Job drawing, mm, ordinate dimensions from the low corner. One solid piece. Round coordinates to 2 decimals unless told otherwise and drop trailing zeros. Write each loop counter-clockwise with the first axis right and the second up, starting at its lowest first coordinate (ties: lowest second). Pieces come first, ordered by that corner, then holes.
1) Saw through at D-D (z = 3). Write the cut outline in (x, y) (3 decimals), plus the area to 3 significant figures.
2) Wall check: probe 1 along Y at (x, z) = (1.25, 25.4) (1 decimal); probe 2 along Y at (x, z) = (0.7, 30) (3 decimals); probe 3 along Y at (x, z) = (0.95, 48). Give the ranges that are in metal, low to high.
3) Saw through at C-C (y = 25.4). Write the cut outline in (x, z) (1 decimal).
4) Saw through at A-A (z = 25.4). Write the cut outline in (x, y) (1 decimal).
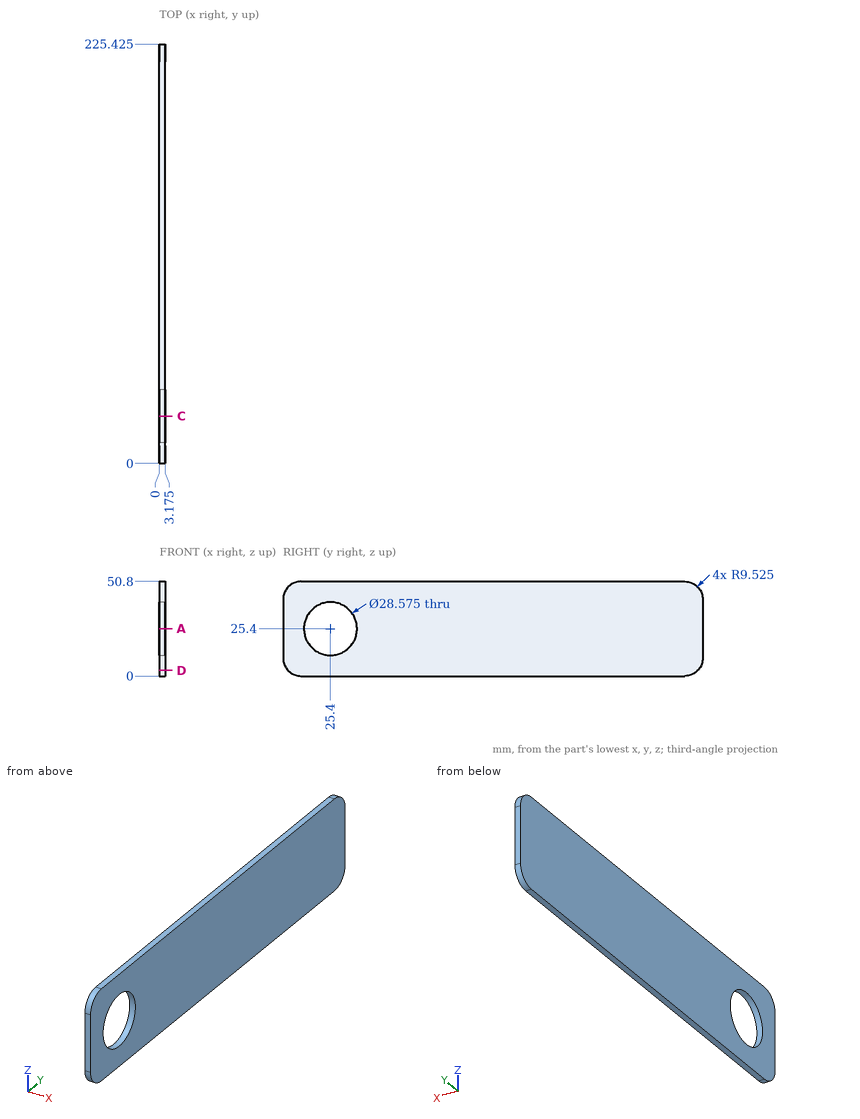
Evaluation:
1. outline: (0, 2.586) - (3.175, 2.586) - (3.175, 222.839) - (0, 222.839) - close
1. area: 699 mm2
2. probe 1: y = 0 to 11.1, 39.7 to 225.4
2. probe 2: y = 0 to 11.873, 38.927 to 225.425
2. probe 3: y = 2.78 to 222.65
3. outline: (0, 0) - (3.2, 0) - (3.2, 11.1) - (0, 11.1) - close; (0, 39.7) - (3.2, 39.7) - (3.2, 50.8) - (0, 50.8) - close
4. outline: (0, 0) - (3.2, 0) - (3.2, 11.1) - (0, 11.1) - close; (0, 39.7) - (3.2, 39.7) - (3.2, 225.4) - (0, 225.4) - close
